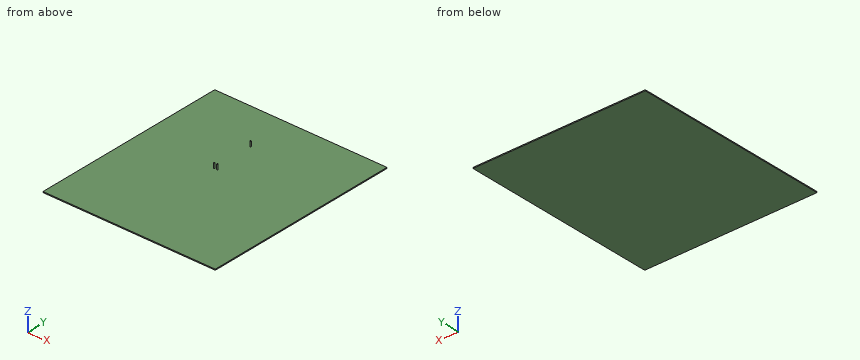
```python
from build123d import *

# Parameters (mm, degrees)
ESBO_O1_W                = 350
ESBO_O1_H                = 400
RESSALTO_EXTRUS_O1_DEPTH = 2
ESBO_O2_R                = 1
RESSALTO_EXTRUS_O2_DEPTH = 10


with BuildPart() as part:
    # Esboço1 → Ressalto-extrusão1 (new body)
    with BuildSketch(Plane.XY):
        Rectangle(ESBO_O1_W, ESBO_O1_H)
    extrude(amount=RESSALTO_EXTRUS_O1_DEPTH)

    # Esboço2 → Ressalto-extrusão2 (add)
    with BuildSketch(Plane.XY.offset(2)):
        with Locations(Location((-16.6, 24.5, 0), (0, 0, 180))):
            Circle(ESBO_O2_R)
        with Locations(Location((-22.77, 24.27, 0), (0, 0, 180))):
            Circle(ESBO_O2_R)
        with Locations(Location((-22.83, 109.16, 0), (0, 0, 180))):
            Circle(ESBO_O2_R)
    extrude(amount=RESSALTO_EXTRUS_O2_DEPTH)


solid = part.part
```
Geometry: final body of the model. Coordinates: model frame, mm. Round coordinates to 2 decimals unless told otherwise and drop trailing zeros. Order: outer loops, then holes, each group sorted by start corner. A loop starts at its lowest first (then second) coordinate and runs counter-clockwise, first axis right, second up. Notation, with made-up numbers: (70.25, -10) - (84.25, -10) arc R24 ccw to (84.25, 25) - close; hole circle Ø8 at (56, 0.25). An arc over 180 degrees is marked (long way). Write item = value, one per line. Start each with the question number.
Q1. Cut plane B-B on y = 170. Return the cut outline in (x, z), and give its area (3 significant figures).
Q2. Ray query, line 1 (Z direction, x = -40.5, y = 72). Return the intervals inside material, ascending. Write a range as from..to.
Q3. Pin query (flat end, axial travel): pin 1 (1.5 mm diameter, centred on x = -106, y = -15.5, fed in from +Z); pin 2 (1.5 mm diameter, centred on x = 96, y = 51.5, fed in from -Z); pin 3 (6 mm diameter, centred on y = -108, z = 5.5, fed in from -X). Return the tip coordinate at first contact, or that it passes through.
Q4. Cut plane A-A on z = 6. Return the cut outline in (x, y).
Q5. Cut plane C-C on x = 127. Return the cut outline in (y, z).
Outcome:
q1.outline = (-175, 0) - (175, 0) - (175, 2) - (-175, 2) - close
q1.area = 700 mm^2
q2.line_1 = 0..2
q3.pin_1 = 2
q3.pin_2 = 0
q3.pin_3 = through
q4.outline = circle Ø2 at (-22.83, 109.16); circle Ø2 at (-22.77, 24.27); circle Ø2 at (-16.6, 24.5)
q5.outline = (-200, 0) - (200, 0) - (200, 2) - (-200, 2) - close
